Answer from the drawing. Dimensions are ordinates in mm from the lowest x, y and z of the part. Round coordinates to 2 decimals unless told otherwise and drop trailing zeros. Loops run counter-clockwise (first coordinate to the right, second up) from the corner with the lowest first, then second, coordinate; pieces in that order, holes last. Notation, with made-up numbers: (50.25, 76) -> (72.25, 76) arc R10 ccw to (72.25, 83) -> close; hole circle Ø5 at (4.25, -19.5). An arc over 180 degrees is marked (long way). Use CSV: the item, a comma, the result in double quotes. Start each with the question number.
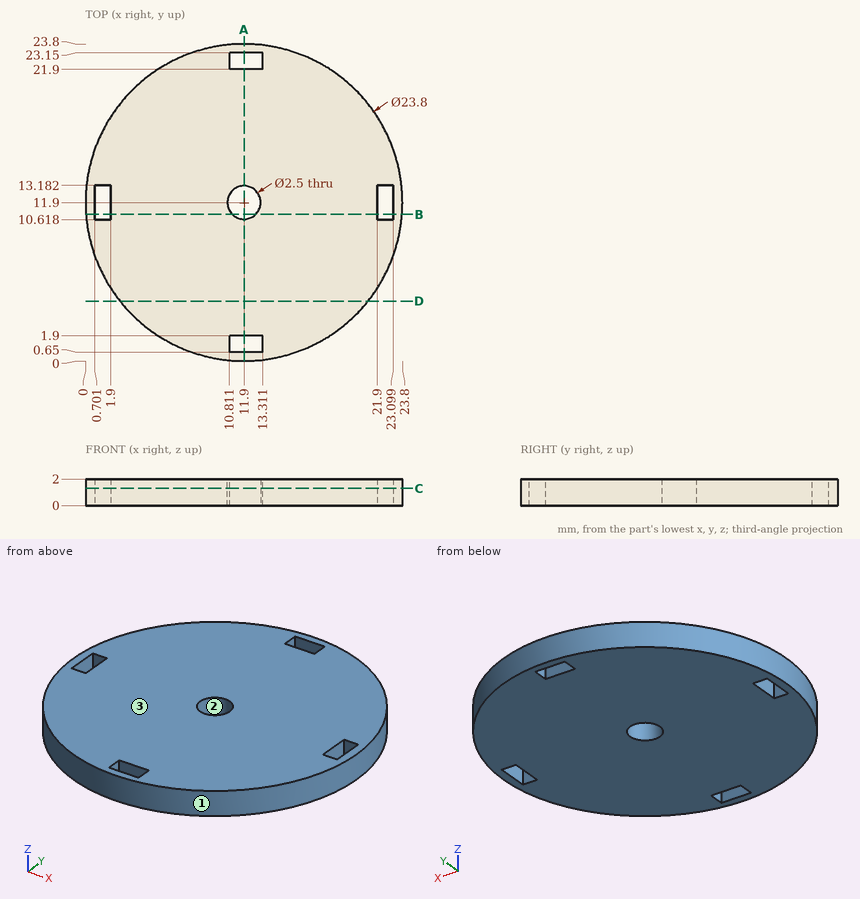
Q1. Straight lines are drawn through the part: line 1 (Y direction, x = 11.9, z = 1.35); line 2 (X direction, y = 12, z = 1.75) (1 decimal); line 3 (Y direction, x = 5.5, z = 0.95). For each, find the intervals that lie inside material, in ascending order. Write a range as from..to.
Q2. Each of these flat-tipped pins is pushed along its axis until it touches: pin 1 (0.6 mm diameter, centred on x = 22.5, z = 1, fed in from +Y); pin 2 (1 mm diameter, centred on y = 1, z = 1.5, fed in from +X) (1 decimal); pin 3 (1 mm diameter, centred on y = 19.5, z = 0.5, fed in from +X). Where does it stop, or does it pass through?
Q3. For a pull along Y with two mould halves and no side action, classify the marked faces 1, 2 and 3 as pulls with the +Y half, pulls with the -Y half, needs draft (parallel to the pull), parting line crosses it, or undercut.
Q4. Section B-B, the plane y = 11 is taken. Write down the section's boundary in (x, z) (1 decimal).
Q5. Section A-A, the plane x = 11.9 is taken. Write down the section's boundary in (y, z).
Q6. Section C-C, the plane z = 1.3 is taken. Write down the section's boundary in (x, y).
Q7. Section D-D, the plane y = 4.5 is taken. Write down the section's boundary in (x, z).
Report:
1,line 1,"y = 0..0.65, 1.9..10.65, 13.15..21.9, 23.15..23.8"
1,line 2,"x = 0..0.7, 1.9..10.7, 13.1..21.9, 23.1..23.8"
1,line 3,"y = 1.87..21.93"
2,pin 1,"stops at y = 17.86"
2,pin 2,"stops at x = 17.7"
2,pin 3,"stops at x = 21.45"
3,face 1,"parting line crosses it"
3,face 2,"undercut"
3,face 3,"needs draft"
4,outline,"(0, 0) -> (0.7, 0) -> (0.7, 2) -> (0, 2) -> close; (1.9, 0) -> (11, 0) -> (11, 2) -> (1.9, 2) -> close; (12.8, 0) -> (21.9, 0) -> (21.9, 2) -> (12.8, 2) -> close; (23.1, 0) -> (23.8, 0) -> (23.8, 2) -> (23.1, 2) -> close"
5,outline,"(0, 0) -> (0.65, 0) -> (0.65, 2) -> (0, 2) -> close; (1.9, 0) -> (10.65, 0) -> (10.65, 2) -> (1.9, 2) -> close; (13.15, 0) -> (21.9, 0) -> (21.9, 2) -> (13.15, 2) -> close; (23.15, 0) -> (23.8, 0) -> (23.8, 2) -> (23.15, 2) -> close"
6,outline,"circle Ø23.8 at (11.9, 11.9); hole (0.7, 10.62) -> (1.9, 10.62) -> (1.9, 13.18) -> (0.7, 13.18) -> close; hole circle Ø2.5 at (11.9, 11.9); hole (10.81, 0.65) -> (13.31, 0.65) -> (13.31, 1.9) -> (10.81, 1.9) -> close; hole (10.81, 21.9) -> (13.31, 21.9) -> (13.31, 23.15) -> (10.81, 23.15) -> close; hole (21.9, 10.62) -> (23.1, 10.62) -> (23.1, 13.18) -> (21.9, 13.18) -> close"
7,outline,"(2.58, 0) -> (21.22, 0) -> (21.22, 2) -> (2.58, 2) -> close"
